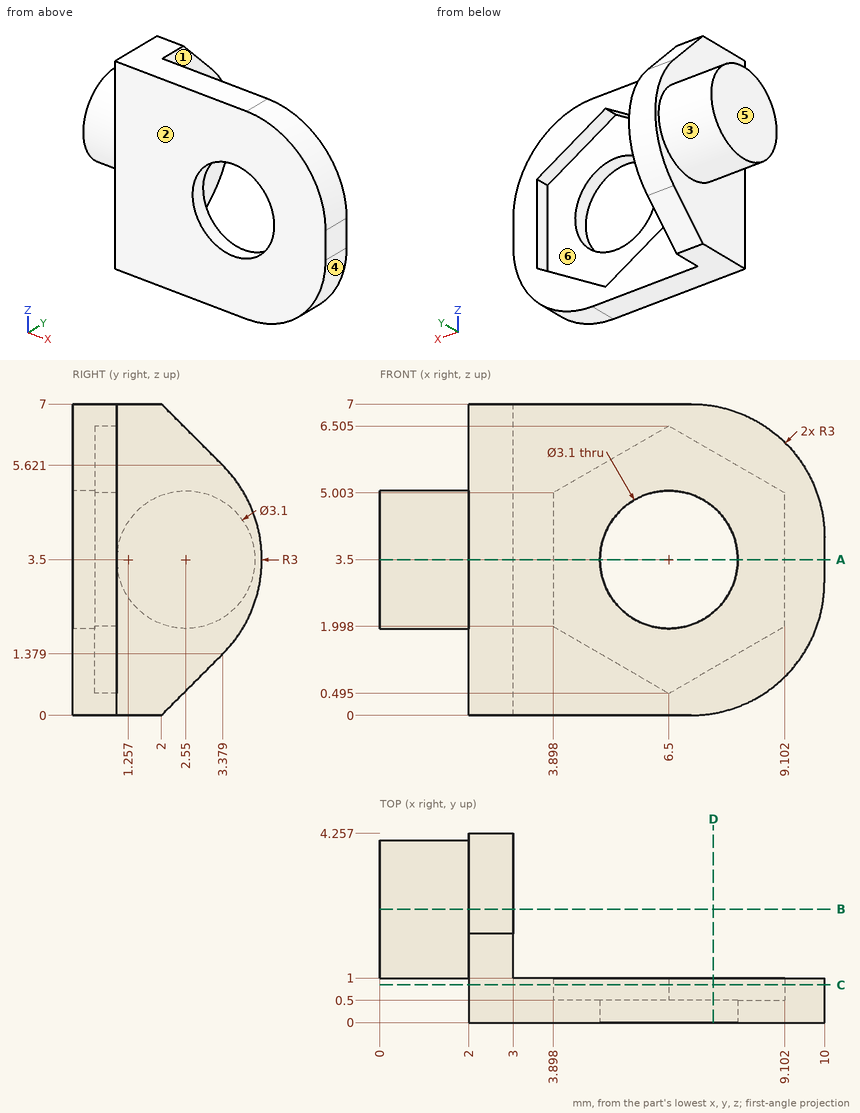
The figure shows three views and two pictorial views of one solid part (mm, origin at its lowest corner). Answer the questions. A direction names the side the tool comes from. Round coordinates to 2 decimals unless told otherwise and drop trailing zeros. Write each loop counter-clockwise with the first axis right and the second up, starting at its lowest first coordinate (ties: lowest second). Pieces come first, ordered by that corner, then holes. Notation, with made-up numbers: (-3, 64) - (9, 64) arc R27 cw to (9, 82) - close; hole circle Ø5 at (86, 79.5). An arc over 180 degrees is marked (long way). One line per question, with ' | ' between items. Start each with the question number.
1. Section A-A (z = 3.5) is taken. Determine the outline of the cut face in (x, y).
2. Section D-D (x = 7.5) is taken. Determine the outline of the cut face in (y, z) (1 decimal).
3. Section C-C (y = 0.85) is taken. Determine the outline of the cut face in (x, z) (1 decimal).
4. For a pull along Z with two mould halves and no side action, classify the marked faces 3, 4, 5 and 6 as +Z half, -Z half, draft (parallel to the pull), parting line (faces both ways), or undercut.
5. Each of these flat-tipped pins is pushed along its axis until it touches: pin 1 (3 mm diameter, centred on x = 6.5, z = 3.5, fed in from -Y) (3 decimals); pin 2 (3 mm diameter, centred on x = 7, z = 5, fed in from +Y); pin 3 (1.5 mm diameter, centred on y = 1.5, z = 1.5, fed in from +X); pin 4 (1.5 mm diameter, centred on y = 3.5, z = 1.5, fed in from +X). Where does it stop, or does it pass through?
6. Section B-B (y = 2.55) is taken. Determine the outline of the cut face in (x, z).
7. Find the intervals of material crossed by probe 1 along Z at (x, y) = (6.5, 0.2); probe 2 along X at (y, z) = (0.1, 3.5); probe 3 along X at (y, z) = (0.85, 3), in increasing order. Write a range as [from, to].
8. For the marked faces 1 and 2, determine the directions among +Z, -Z, +X, -X, +Y, -Y from which every point of the face is accessible in a straight line to the end or side of a thin tool.
Filled in:
1) outline: (0, 1) - (2, 1) - (2, 0) - (4.95, 0) - (4.95, 0.5) - (3.9, 0.5) - (3.9, 1) - (3, 1) - (3, 4.26) - (2, 4.26) - (2, 4.1) - (0, 4.1) - close; (8.05, 0) - (10, 0) - (10, 1) - (9.1, 1) - (9.1, 0.5) - (8.05, 0.5) - close
2) outline: (0, 0) - (1, 0) - (1, 1.1) - (0.5, 1.1) - (0.5, 2.3) - (0, 2.3) - close; (0, 4.7) - (0.5, 4.7) - (0.5, 5.9) - (1, 5.9) - (1, 7) - (0, 7) - close
3) outline: (2, 0) - (7, 0) arc R3 ccw to (10, 3) - (10, 4) arc R3 ccw to (7, 7) - (2, 7) - close; hole (3.9, 2) - (6.5, 0.5) - (9.1, 2) - (9.1, 5) - (6.5, 6.5) - (3.9, 5) - close
4) face 3: parting line | face 4: -Z half | face 5: draft | face 6: undercut
5) pin 1: through | pin 2: y = 1 | pin 3: x = 9.85 | pin 4: x = 3
6) outline: (0, 1.95) - (2, 1.95) - (2, 0.55) - (3, 0.55) - (3, 6.45) - (2, 6.45) - (2, 5.05) - (0, 5.05) - close
7) probe 1: [0, 1.95], [5.05, 7] | probe 2: [2, 4.95], [8.05, 10] | probe 3: [2, 3.9], [9.1, 10]
8) face 1: +Z, -Z, +X, +Y | face 2: +Z, -Z, +X, -X, -Y
